```python
from build123d import *

# Parameters (mm, degrees)
F0_W       = 91.4399989891
F0_H       = 99.0599989891
F0_W_2     = 81.28
F0_H_2     = 88.9
F1_DEPTH   = 17.78
F2_W       = 91.4399989891
F2_H       = 99.0599989891
F3_DEPTH   = 5.08
F4_SIZE    = 5.08
F6_DEPTH   = 25.4
F7_R       = 2.286
F8_DEPTH   = 25.4
F10_DEPTH  = 2.54
F11_SIZE   = 5.07999
F11_SIZE_2 = 5.08
F13_DEPTH  = 50.8


# Not quite as in the source:
# - a fillet or chamfer is up to 0.001 mm smaller than in the source, because OpenCascade refuses the exact size


with BuildPart() as f1:
    # F0 (on Top) → F1 (new body)
    with BuildSketch(Plane.XY):
        Rectangle(F0_W, F0_H)
        Rectangle(F0_W_2, F0_H_2, mode=Mode.SUBTRACT)
    extrude(amount=-F1_DEPTH)

    # F2 (on face) → F3 (join)
    with BuildSketch(Plane.XY):
        Rectangle(F2_W, F2_H)
    extrude(amount=F3_DEPTH)

    # F4
    f4_edges = [f1.edges().sort_by_distance(p)[0] for p in [
        (-45.719999, 49.529999, -6.35),
        (45.719999, 49.529999, -6.35),
        (45.719999, -49.529999, -6.35),
        (-45.719999, -49.529999, -6.35),
    ]]
    chamfer(f4_edges, length=F4_SIZE)

    # F5 (on Front) → F6 (join, symmetric)
    with BuildSketch(Plane.XZ):
        Polygon((10.8585, 7.5946), (8.3439, 5.08), (15.875, 5.08), (15.875, 14.4018), (8.3439, 14.4018), (8.3439, 10.1092), align=None)
        Polygon((-8.3439, 10.1092), (-8.3439, 14.4018), (-15.875, 14.4018), (-15.875, 5.08), (-8.3439, 5.08), (-10.8585, 7.5946), align=None)
    extrude(amount=F6_DEPTH, both=True)

    # F7 (on face) → F8 (cut)
    with BuildSketch(Plane(origin=(0, 0, 0), x_dir=(1, 0, 0), z_dir=(0, 0, -1))):
        Circle(F7_R)
    extrude(amount=-F8_DEPTH, mode=Mode.SUBTRACT)

    # F9 (on face) → F10 (cut)
    with BuildSketch(Plane.XY.offset(5.08)):
        Polygon((2.5204947689, 4.365625), (-2.5204947689, 4.365625), (-5.0409895379, 0), (-2.5204947689, -4.365625), (2.5204947689, -4.365625), (5.0409895379, 0), align=None)
    extrude(amount=-F10_DEPTH, mode=Mode.SUBTRACT)

    # F11 (call 1 of 8: OpenCascade refuses the feature's edges together) (size 5.08 in the source; OpenCascade refuses exactly that, so slightly less here)
    f11_edges = [f1.edges().sort_by_distance(p)[0] for p in [
        (0, 49.529999, -17.78),
    ]]
    chamfer(f11_edges, length=F11_SIZE)

    # F11#2 (call 2 of 8) (size 5.08 in the source; OpenCascade refuses exactly that, so slightly less here)
    f11_2_edges = [f1.edges().sort_by_distance(p)[0] for p in [
        (-45.719999, 0, -17.78),
    ]]
    chamfer(f11_2_edges, length=F11_SIZE)

    # F11#3 (call 3 of 8) (size 5.08 in the source; OpenCascade refuses exactly that, so slightly less here)
    f11_3_edges = [f1.edges().sort_by_distance(p)[0] for p in [
        (0, -49.529999, -17.78),
    ]]
    chamfer(f11_3_edges, length=F11_SIZE)

    # F11#4 (call 4 of 8) (size 5.08 in the source; OpenCascade refuses exactly that, so slightly less here)
    f11_4_edges = [f1.edges().sort_by_distance(p)[0] for p in [
        (45.719999, 0, -17.78),
    ]]
    chamfer(f11_4_edges, length=F11_SIZE)

    # F11#5 (call 5 of 8)
    f11_5_edges = [f1.edges().sort_by_distance(p)[0] for p in [
        (0, 49.529999, 5.08),
    ]]
    chamfer(f11_5_edges, length=F11_SIZE_2)

    # F11#6 (call 6 of 8)
    f11_6_edges = [f1.edges().sort_by_distance(p)[0] for p in [
        (-45.719999, 0, 5.08),
    ]]
    chamfer(f11_6_edges, length=F11_SIZE_2)

    # F11#7 (call 7 of 8)
    f11_7_edges = [f1.edges().sort_by_distance(p)[0] for p in [
        (0, -49.529999, 5.08),
    ]]
    chamfer(f11_7_edges, length=F11_SIZE_2)

    # F11#8 (call 8 of 8)
    f11_8_edges = [f1.edges().sort_by_distance(p)[0] for p in [
        (45.719999, 0, 5.08),
    ]]
    chamfer(f11_8_edges, length=F11_SIZE_2)

    # F12 (on face) → F13 (join, through all)
    with BuildSketch(Plane.XZ.offset(25.4)):
        Polygon((-15.875, 14.4018), (-23.495, 5.08), (-15.875, 5.08), align=None)
        Polygon((23.495, 5.08), (15.875, 14.4018), (15.875, 5.08), align=None)
    extrude(amount=-F13_DEPTH)


solid = f1.part
```
Could you check a few things on this model? Use its own coordinates, in mm. A direction names the side the tool comes from. Coordinates: 2 decimals unless noted, no trailing zeros. Write each loop counter-clockwise with the first axis right and the second up, starting at its lowest first coordinate (ties: lowest second). Pieces come first, ordered by that corner, then holes. Notation, with made-up numbers: (27, 22.25) -> (58, 22.25) arc R26 cw to (58, 47.25) -> close; hole circle Ø7 at (43, -7.75). An arc over 180 degrees is marked (long way). Return JSON: item names as keys, results as strings.
(1) Which directions (+Z, -Z, +X, -X, +Y, -Y) give clear straight access to the entire face, cutting with the end or side of a thin tool? Please do faces 4 (the flat face through (8.344, 0, 12)), 5 (the flat face through (43.22, -0.66, 2.5)), 6 (the flat face through (3.8, 2.15, 3.83)), 7 (the flat face through (40.64, -1, -9)).
Numbers:
{"face 4": "+Z, +Y, -Y", "face 5": "+Z, +X, +Y, -Y", "face 6": "+Z", "face 7": "-Z"}
(2) I'm going to push flat-ended pins straight in: pin 1 (10.5 mm diameter, centred on x = -18, z = 9.5, fed in from +Y); pin 2 (0.8 mm diameter, centred on x = 0, z = 3.5, fed in from -Y); pin 3 (3.5 mm diameter, centred on x = 0, y = 0, fed in from +Z); pin 4 (10 mm diameter, centred on x = -5, y = -39.5, fed in from -Z). Where does each tip first touch, or does it pass through?
Numbers:
{"pin 1": "stops at y = 45.28", "pin 2": "stops at y = -46.43", "pin 3": "passes through", "pin 4": "stops at z = -17.78"}
(3) Imagine slicing it at B-B, the plane z = -9. Please give me the cut outline in (x, y), then the cut area to 3 significant figures.
Numbers:
{"outline": "(-45.72, -44.45) -> (-40.64, -49.53) -> (40.64, -49.53) -> (45.72, -44.45) -> (45.72, 44.45) -> (40.64, 49.53) -> (-40.64, 49.53) -> (-45.72, 44.45) -> close; hole (-40.64, -44.45) -> (40.64, -44.45) -> (40.64, 44.45) -> (-40.64, 44.45) -> close", "area": "1,780 mm2"}
(4) We'd pull the mould along X, two halves only. Please class faces 1 (the flat face through (-9.619, -0.356, 8.834)), 2 (the flat face through (-19.63, -0.36, 9.81)), 3 (the flat face through (-14, 25.4, 10)): +X half, -X half, draft (parallel to the pull), parting line (faces both ways), or undercut.
Numbers:
{"face 1": "undercut", "face 2": "-X half", "face 3": "draft"}
(5) I need wall thicknesses on L1, parallel to Y at x = -16, z = -5.5; L2, parallel to X at y = -20, z = -5; L3, parallel to Z at x = -12, y = 25.5. Which ranges of each line are inside material? Lowest first, please.
Numbers:
{"L1": "y = -49.53 to -44.45, 44.45 to 49.53", "L2": "x = -45.72 to -40.64, 40.64 to 45.72", "L3": "z = 0 to 5.08"}
